Read the model definition and answer for the solid it produces. Units are mm, in the model's axes. Face numbers are marked on the shaded views. A direction names the side the tool comes from. Coordinates: 2 decimals unless noted, no trailing zeros. Order: outer loops, then holes, each group sorted by start corner. A loop starts at its lowest first (then second) coordinate and runs counter-clockwise, first axis right, second up. Notation, with made-up numbers: (27, 33.25) -> (42, 33.25) arc R4 ccw to (42, 37.25) -> close; hole circle Ø2 at (-20.75, 45). An arc over 180 degrees is marked (long way). Answer as a JSON object with one key per item and string values. Group by question number.
1) Consider L1, parallel to X at y = 11.5, z = 9; L2, parallel to Y at x = -7.5, z = 26.5 (3 decimals); L3, parallel to Y at x = 5.5, z = 16.5. Determine where each line is inside the solid, lowest interval first.
2) A tool of negligible diameter and unlimited length cuts with its end or side. For the marked faces 4, 5, 6 and 7, from which of +Z, -Z, +X, -X, +Y, -Y can it reach the whole face along a straight path? Write none if from no direction.
3) Section C-C on y = 9.5 is taken. Determine the outline of the cut face in (x, z) (1 decimal), and give its area (3 significant figures).
4) Section A-A on x = -2.75 is taken. Determine the outline of the cut face in (y, z) (3 decimals), and give its area (3 significant figures).
5) Determine the mould class of the marked faces 1, 2 and 3 for opening direction Y: released by +Y, released by -Y, zero draft, split by the parting line, or undercut.
6) Section B-B on z = 0 is taken. Determine the outline of the cut face in (x, y).
7) Given pin 1 (4.5 mm diameter, centred on x = 3, z = 25.5, fed in from +Y); pin 2 (1.4 mm diameter, centred on x = -1.5, z = 12.5, fed in from -Y); pin 3 (6 mm diameter, centred on y = 32, z = 19.5, fed in from -X); pin 4 (1 mm diameter, centred on x = 4, y = 44, fed in from +Z), each flat-ended and moving along its own axis, determine where each tip first touches the part or whether it passes through.
8) Section D-D on x = 0.75 is taken. Determine the outline of the cut face in (y, z) (3 decimals), and give its area (3 significant figures).
Autodesk Inventor part; units mm, degrees
ref_plane "YZ Plane" through (0, 0, 0) normal (1, 0, 0) x (0, 1, 0)
ref_plane "XZ Plane" through (0, 0, 0) normal (0, 1, 0) x (-1, 0, 0)
ref_plane "XY Plane" through (0, 0, 0) normal (0, 0, 1) x (1, 0, 0)
sketch "Sketch1" plane through (0, 0, 0) normal (1, 0, 0) x (0, 1, 0)
  arc A0 (39.954, 1.6866) -> (44.513, 5.9979) centre (40.195, 5.9979) ccw
  circle A1 centre (40.195, 5.9979) radius 1.5875
  line L0 (44.513, 5.9979) -> (44.513, 20.9839)
  line L1 (44.513, 20.9839) -> (42.481, 20.9839)
  line L2 (42.481, 20.9839) -> (42.481, 27.5879)
  line L3 (42.481, 27.5879) -> (38.417, 27.5879)
  line L4 (38.417, 27.5879) -> (38.417, 23.5239)
  line L5 (39.954, 1.6866) -> (37.414, 1.6866)
  line L6 (37.414, 1.6866) -> (36.4393, -3.299)
  line L7 (36.4393, -3.299) -> (10.8933, -7.6145)
  line L8 (10.8933, -7.6145) -> (7.2025, -0.948)
  line L9 (7.2025, -0.948) -> (2.0915, -3.7777)
  arc A2 (-3.6468, 2.3121) -> (2.0915, -3.7777) centre (0, 0) ccw
  circle A3 centre (0, 0) radius 1.5875
  line L10 (8.191, 27.5879) -> (12.255, 27.5879)
  line L11 (12.255, 27.5879) -> (12.255, 23.5239)
  arc A4 (12.255, 23.5239) -> (38.417, 23.5239) centre (25.336, 23.5239) ccw
  line L12 (81.5814, 1.6799) -> (58.7298, 1.6799) construction
  line L13 (40.195, 5.9979) -> (0, 0) construction
  line L14 (8.191, 27.5879) -> (10.8933, -7.6145) construction
  line L15 (60.3567, 10.4429) -> (44.3212, 10.4429) construction
  line L16 (8.191, 27.5879) -> (0, 0) construction
  line L17 (-6.8832, 3.5179) -> (4.3798, -16.8256) construction
  line L18 (8.191, 27.5879) -> (8.191, 20.9839)
  line L19 (8.191, 20.9839) -> (-3.6468, 2.3121)
  dimension "d0" = 8.636
  dimension "d1" = 3.175
  dimension "d2" = 4.064
  dimension "d3" = 6.604
  dimension "d4" = 2.032
  dimension "d5" = 25.908
  dimension "d6" = 2.54
  dimension "d7" = 5.08
  dimension "d8" = 25.908
  dimension "d9" = 7.62
  dimension "d10" = 40.64
  dimension "d11" = 35.306
  dimension "d12" = 26.162
  dimension "d13" = 17.145
  dimension "d14" = 28.7782
  dimension "d15" = 10.16
extrude "Extrusion1" add sketch "Sketch1" along normal mid plane 16.002
sketch "Sketch2" plane through (0, 0, 0) normal (1, 0, 0) x (0, 1, 0)
  line L0 (38.417, 27.5879) -> (42.481, 27.5879)
  line L1 (8.191, 27.5879) -> (12.255, 27.5879)
  line L2 (41.338, 10.4429) -> (11.366, 10.4429)
  line L3 (44.513, 20.9839) -> (44.513, 5.9979)
  arc A0 (41.338, 10.4429) -> (44.513, 13.6179) centre (41.338, 13.6179) ccw
  line L4 (8.191, 27.5879) -> (8.191, 13.6179)
  arc A1 (8.191, 13.6179) -> (11.366, 10.4429) centre (11.366, 13.6179) ccw
  line L5 (44.513, 13.6179) -> (46.9295, 13.6179)
  line L6 (46.9295, 13.6179) -> (49.0826, -15.2272)
  line L7 (49.0826, -15.2272) -> (-26.66, -17.9242)
  line L8 (-26.66, -17.9242) -> (-26.66, 23.5652)
  line L9 (-26.66, 23.5652) -> (8.191, 27.5879)
  point P0 (0, 0)
  point P1 (44.513, 3.2824)
  dimension "d18" = 17.145
  dimension "d19" = 3.175
  dimension "d20" = 3.175
extrude "Extrusion2" cut sketch "Sketch2" along normal mid plane 10.16
sketch "Sketch3" plane through (-8.001, 38.417, 27.5879) normal (0, 0, 1) x (1, 0, 0)
  line L0 (16.002, -26.162) -> (0, -26.162)
  line L1 (16.002, -30.226) -> (0, -30.226)
  line L2 (0, -30.226) -> (0, -26.162)
  line L3 (16.002, -26.162) -> (16.002, -30.226)
  line L4 (0, 4.064) -> (16.002, -30.226) construction
  line L5 (4.572, -3.175) -> (11.43, -3.175)
  line L6 (11.43, -3.175) -> (11.43, -22.987)
  line L7 (11.43, -22.987) -> (4.572, -22.987)
  line L8 (4.572, -22.987) -> (4.572, -3.175)
  line L9 (11.43, -3.175) -> (4.572, -22.987) construction
  point P0 (8.001, -38.417)
  point P1 (8.001, -13.081)
  dimension "d23" = 6.858
  dimension "d24" = 19.812
extrude "Extrusion3" cut sketch "Sketch3" against normal through all contours L5 L6 L7 L8
sketch "Sketch4" plane through (-8.001, 42.481, 27.5879) normal (0, 1, 0) x (1, 0, 0)
  line L0 (16.002, 0) -> (0, 0)
  circle A0 centre (8.362, 4.064) radius 1.5875
  point P0 (8.001, 27.5879)
  dimension "d27" = 3.175
  dimension "d28" = 4.064
extrude "Extrusion4" cut sketch "Sketch4" against normal through all
properties part number "Front Axle Housing" material "ABS Plastic"
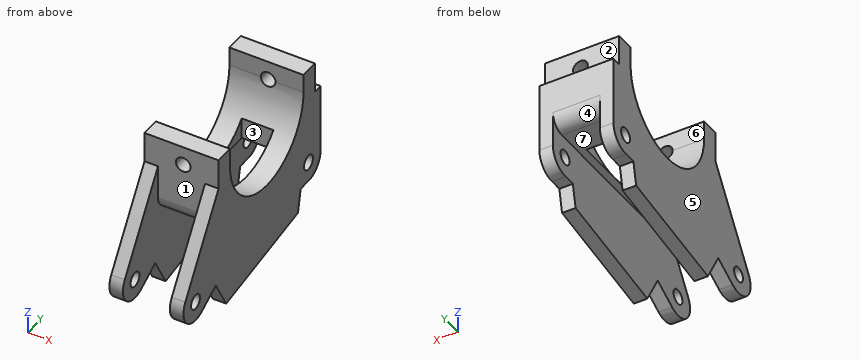
Worked answers:
{
 "1": {"L1": "x = -8 to -5.08, 5.08 to 8", "L2": "y = 8.191 to 12.255, 38.417 to 42.481", "L3": "y = 5.35 to 14.3, 36.37 to 44.51"},
 "2": {"face 4": "-Z, +Y", "face 5": "+Z, -Z, -X, +Y, -Y", "face 6": "+Z, +X, -X", "face 7": "-Z, +Y, -Y"},
 "3": {"outline": "(-8, -5.1) -> (-5.1, -5.1) -> (-5.1, 11) -> (5.1, 11) -> (5.1, -5.1) -> (8, -5.1) -> (8, 27.6) -> (-8, 27.6) -> close; hole circle Ø3.2 at (0.4, 23.5)", "area": "351 mm²"},
 "4": {"outline": "(8.191, 13.618) arc R3.175 ccw to (11.366, 10.443) -> (15.43, 10.443) -> (15.43, 14.981) arc R13.081 cw to (12.255, 23.524) -> (12.255, 27.588) -> (8.191, 27.588) -> close; (35.242, 10.443) -> (41.338, 10.443) arc R3.175 ccw to (44.513, 13.618) -> (44.513, 20.984) -> (42.481, 20.984) -> (42.481, 27.588) -> (38.417, 27.588) -> (38.417, 23.524) arc R13.081 cw to (35.242, 14.981) -> close", "area": "202 mm²"},
 "5": {"face 1": "released by -Y", "face 2": "released by +Y", "face 3": "undercut"},
 "6": {"outline": "(-8, -4.32) -> (-5.08, -4.32) -> (-5.08, -1.59) -> (-8, -1.59) -> close; (-8, 1.59) -> (-5.08, 1.59) -> (-5.08, 37.08) -> (-8, 37.08) -> close; (5.08, -4.32) -> (8, -4.32) -> (8, -1.59) -> (5.08, -1.59) -> close; (5.08, 1.59) -> (8, 1.59) -> (8, 37.08) -> (5.08, 37.08) -> close"},
 "7": {"pin 1": "stops at y = 42.48", "pin 2": "stops at y = 8.22", "pin 3": "passes through", "pin 4": "stops at z = 20.98"},
 "8": {"outline": "(8.191, 13.618) arc R3.175 ccw to (11.366, 10.443) -> (15.43, 10.443) -> (15.43, 14.981) arc R13.081 cw to (12.346, 21.985) -> (8.191, 21.985) -> close; (8.191, 25.063) -> (12.255, 25.063) -> (12.255, 27.588) -> (8.191, 27.588) -> close; (35.242, 10.443) -> (41.338, 10.443) arc R3.175 ccw to (44.513, 13.618) -> (44.513, 20.984) -> (42.481, 20.984) -> (42.481, 21.985) -> (38.326, 21.985) arc R13.081 cw to (35.242, 14.981) -> close; (38.417, 25.063) -> (42.481, 25.063) -> (42.481, 27.588) -> (38.417, 27.588) -> close", "area": "177 mm²"}
}
